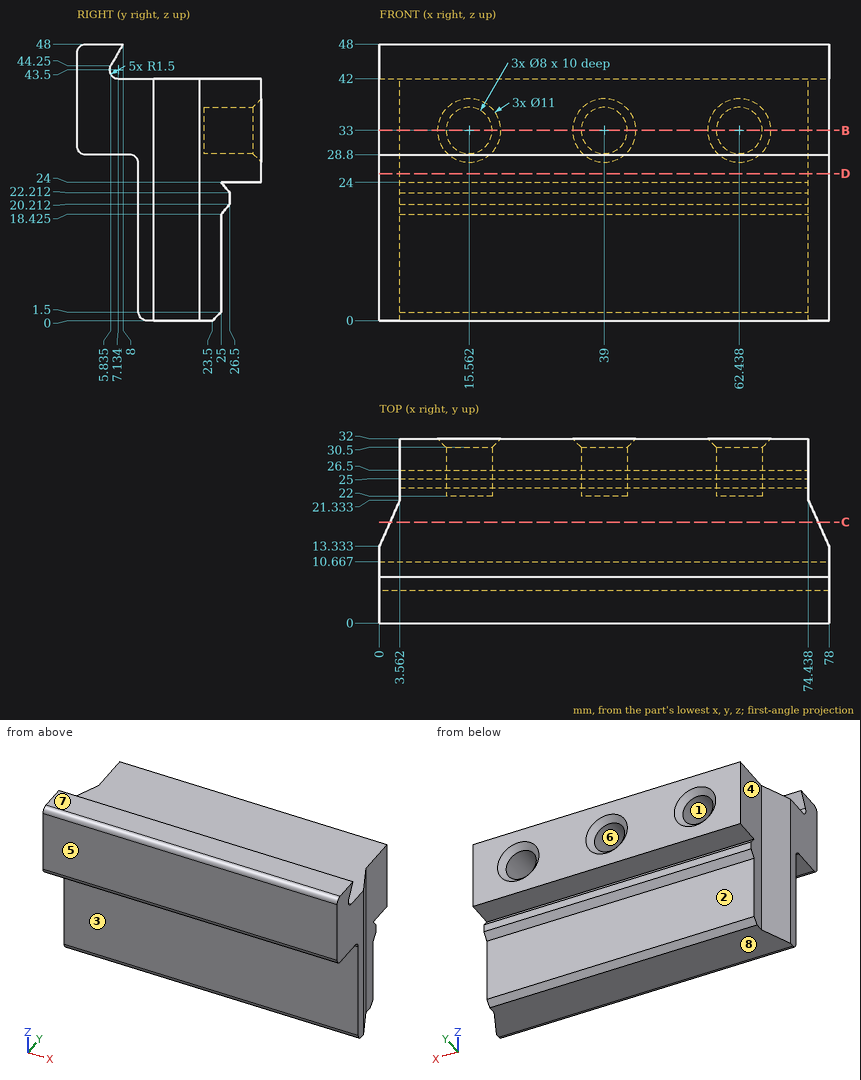
Geometry: see drawing. Coordinates: mm, zero at the bounding-box minimum. A direction names the side the tool comes from. Give positions to 0.01 mm unless a question says otherwise; leave off trailing zeros. Write each loop counter-clockwise with the first axis right and the second up, starting at its lowest first coordinate (ties: lowest second). Pieces come first, ordered by that corner, then holes. Notation, with made-up numbers: (-27, 34) - (-5, 34) arc R17 ccw to (-5, 39) - close; hole circle Ø10 at (-30.5, 24). An arc over 180 degrees is marked (long way). Return JSON: item names as keys, results as strings. Group by question number.
1) Section B-B on z = 33. Return the cut outline in (x, y), plus the area to 3 significant figures.
2) Line query: line 1 (X direction, y = 28, z = 33); line 2 (Z direction, x = 39, y = 27); line 3 (Y direction, x = 36, z = 2). Output: solid intervals per line, ascending.
3) Set-up query: the marked faces 1, 2, 3 and 4. Return all of +Z, -Z, +X, -X, +Y, -Y with unobstructed straight access to the full face (end or side cutting, diameter ignored); none if empty.
4) Section C-C on y = 17.5. Return the cut outline in (x, z) (1 decimal).
5) Section D-D on z = 25.5. Return the cut outline in (x, y), plus the area to 3 significant figures.
6) Mould query, pull axis Z, two halves, no side actions, for the marked faces 5, 6, 7 and 8. Classes: released by +Z, released by -Z, zero draft, split by the parting line, or undercut.
7) First-contact query: P1, Ø12, axis at x = 16, z = 32, coming from the +Y side; P2, Ø1.5, axis at x = 36.5, z = 18.5, coming from the +Y side; P3, Ø6.5, axis at x = 38.5, z = 32, coming from the +Y side; P4, Ø10.5, axis at x = 39, z = 33, coming from the +Y side. Flat tips, straight axial feed; report the tip coordinate or a pass-through.
Filled in:
{
 "1": {"outline": "(0, 0) - (78, 0) - (78, 13.33) - (74.44, 21.33) - (74.44, 32) - (67.94, 32) - (66.44, 30.5) - (66.44, 22) - (58.44, 22) - (58.44, 30.5) - (56.94, 32) - (44.5, 32) - (43, 30.5) - (43, 22) - (35, 22) - (35, 30.5) - (33.5, 32) - (21.06, 32) - (19.56, 30.5) - (19.56, 22) - (11.56, 22) - (11.56, 30.5) - (10.06, 32) - (3.56, 32) - (3.56, 21.33) - (0, 13.33) - close", "area": "2,140 mm^2"},
 "2": {"line 1": "x = 3.56 to 11.56, 19.56 to 35, 43 to 58.44, 66.44 to 74.44", "line 2": "z = 24 to 29, 37 to 42", "line 3": "y = 10.67 to 25"},
 "3": {"face 1": "+Y", "face 2": "-Z, +X, -X, +Y", "face 3": "-Z, +X, -X, -Y", "face 4": "+Z, -Z, -X, +Y"},
 "4": {"outline": "(1.9, 0) - (76.1, 0) - (76.1, 42) - (1.9, 42) - close"},
 "5": {"outline": "(0, 10.67) - (78, 10.67) - (78, 13.33) - (74.44, 21.33) - (74.44, 32) - (3.56, 32) - (3.56, 21.33) - (0, 13.33) - close", "area": "1,560 mm^2"},
 "6": {"face 5": "zero draft", "face 6": "undercut", "face 7": "released by +Z", "face 8": "released by -Z"},
 "7": {"P1": "stops at y = 32", "P2": "stops at y = 25.69", "P3": "stops at y = 30.87", "P4": "stops at y = 31.75"}
}
